Geometry check sheet. Reference: drawing and pictorial views, mm from the part's lowest x, y, z. A direction names the side the tool comes from. Give positions to 0.01 mm unless a question says otherwise; leave off trailing zeros. Write each loop counter-clockwise with the first axis right and the second up, starting at its lowest first coordinate (ties: lowest second). Pieces come first, ordered by that corner, then holes. Notation, with made-up numbers: M -29,2.25 L 30,2.25 A34 cw 30,39.25 Z; hole C 47.25,71.25 d7. An arc over 180 degrees is marked long. One line per item, written item: value. Start each with the question number.
1. Gauge pin test, flat ends, axial feed: pin 1 (10 mm diameter, centred on x = 23, z = 18.5, fed in from +Y); pin 2 (4 mm diameter, centred on x = 24, z = 27, fed in from -Y); pin 3 (1 mm diameter, centred on x = 18.5, y = 56.5, fed in from +Z); pin 4 (12 mm diameter, centred on y = 50, z = 50, fed in from -X). Record the tip position at first contact, or that the pin passes through.
2. Cross-section at B-B on x = 17.5. Record the cut outline in (y, z).
3. Scan lines: line 1 (X direction, y = 62, z = 44.5); line 2 (Z direction, x = 23.25, y = 39.5); line 3 (Z direction, x = 26.25, y = 70). Record each from-to range of solid material in increasing order.
4. Cross-section at A-A on z = 50. Record the cut outline in (x, y).
5. Tool access check on the marked faces 4 and 5. Record the directions out of +Z, -Z, +X, -X, +Y, -Y that give a thin tool (end or side, any length) a straight path to the whole face; none if there is none.
6. Release check for a two-part mould opening along Y. For the marked faces 1, 2 and 3 record: pulls with the +Y half, pulls with the -Y half, needs draft (parallel to the pull), parting line crosses it, or undercut.
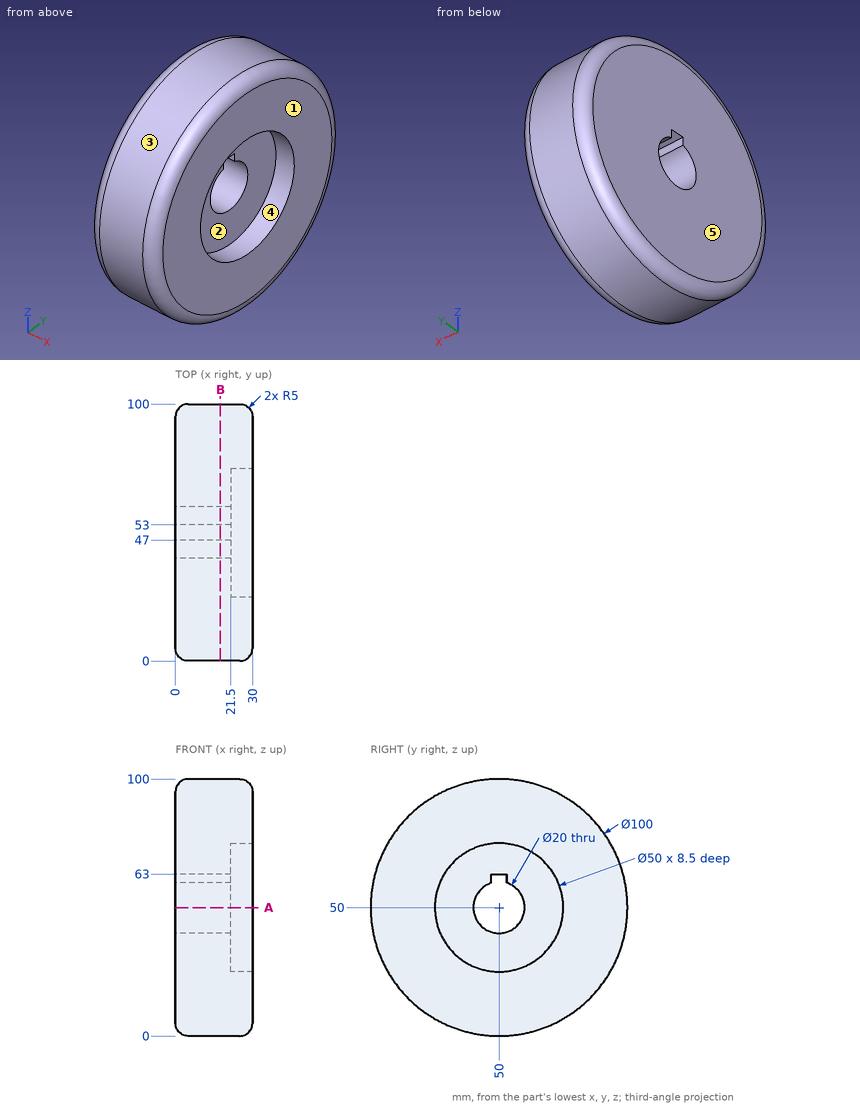
Report:
1. pin 1: stops at y = 92.4
1. pin 2: stops at y = 4.62
1. pin 3: stops at z = 99.64
1. pin 4: passes through
2. outline: C 50,50 d100; hole M 47,59.54 A10 ccw long 53,59.54 L 53,63 L 47,63 Z
3. line 1: x = 0 to 21.5
3. line 2: z = 1.11 to 27.31, 72.69 to 98.89
3. line 3: z = 4.35 to 35, 65 to 95.65
4. outline: M 0,5 A5 ccw 5,0 L 25,0 A5 ccw 30,5 L 30,25 L 21.5,25 L 21.5,40 L 0,40 Z; M 0,60 L 21.5,60 L 21.5,75 L 30,75 L 30,95 A5 ccw 25,100 L 5,100 A5 ccw 0,95 Z
5. face 4: +X
5. face 5: +Z, -Z, -X, +Y, -Y
6. face 1: needs draft
6. face 2: undercut
6. face 3: parting line crosses it
